Job drawing, mm, ordinate dimensions from the low corner. One solid piece. A direction names the side the tool comes from. Give positions to 0.01 mm unless a question says otherwise; leave off trailing zeros. Write each loop counter-clockwise with the first axis right and the second up, starting at its lowest first coordinate (ties: lowest second). Pieces come first, ordered by that corner, then holes. Notation, with made-up numbers: (76.5, 86.25) - (105.5, 86.25) arc R21 ccw to (105.5, 124.25) - close; hole circle Ø10 at (-31.5, 74). An arc over 180 degrees is marked (long way). Answer as a JSON object with one key per item and string values.
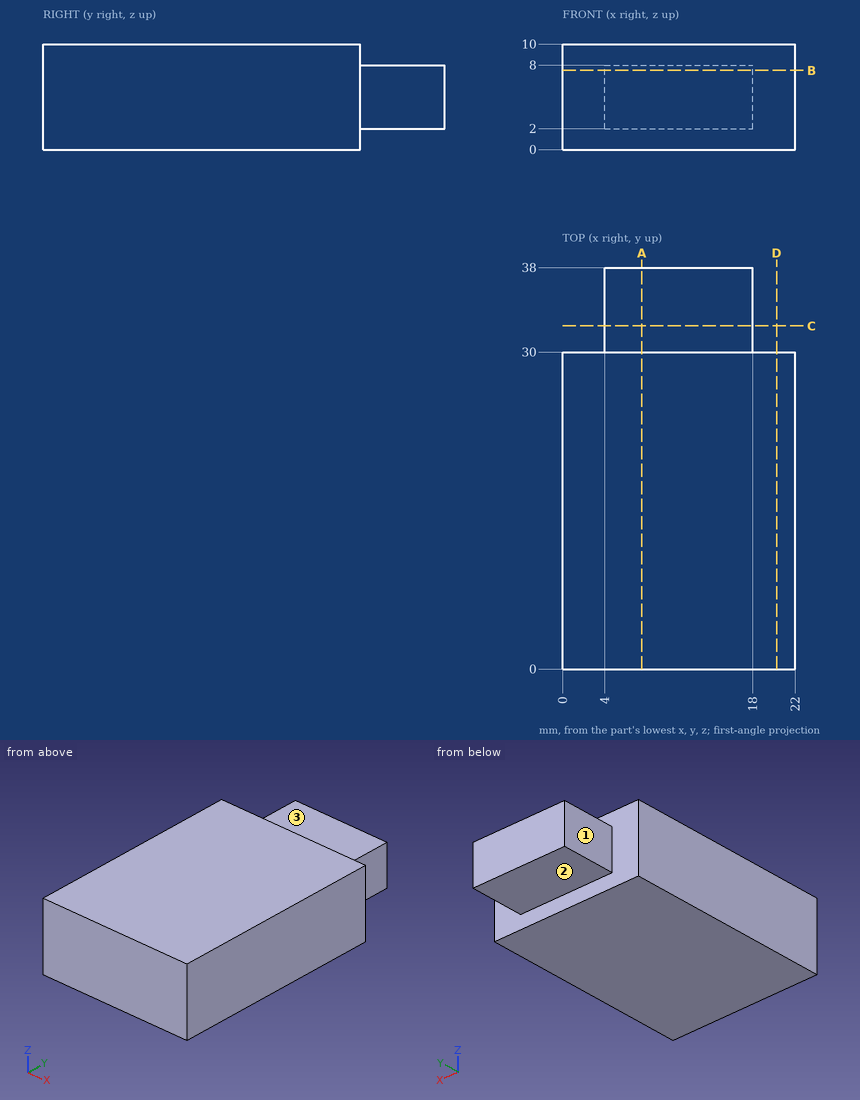
Item 1: Cut at D-D (x = 20.25). Give the cut face in (y, z).
Entries:
{"outline": "(0, 0) - (30, 0) - (30, 10) - (0, 10) - close"}
Item 2: Probe line 1 (Z direction, x = 12, y = 33); line 2 (Y direction, x = 3, z = 3); line 3 (X direction, y = 35, z = 7.75). List the from-to ranges inside material, lowest first. Write a range as from..to.
Entries:
{"line 1": "2..8", "line 2": "0..30", "line 3": "4..18"}
Item 3: Cut at A-A (x = 7.5). Give the cut face in (y, z), and give its area (3 significant figures).
Entries:
{"outline": "(0, 0) - (30, 0) - (30, 2) - (38, 2) - (38, 8) - (30, 8) - (30, 10) - (0, 10) - close", "area": "348 mm2"}
Item 4: Cut at B-B (z = 7.5). Give the cut face in (x, y), and give its area (3 significant figures).
Entries:
{"outline": "(0, 0) - (22, 0) - (22, 30) - (18, 30) - (18, 38) - (4, 38) - (4, 30) - (0, 30) - close", "area": "772 mm2"}
Item 5: Which spindle directions (+Z, -Z, +X, -X, +Y, -Y) get a long thin tool onto all of the face, cutting with end or side? Do the marked faces 1, 2 and 3. Say none if no direction does.
Entries:
{"face 1": "+Z, -Z, -X, +Y", "face 2": "-Z, +X, -X, +Y", "face 3": "+Z, +X, -X, +Y"}
Item 6: Flat gauge pins, fed straight in: P1, Ø3, axis at y = 32.5, z = 3.5, coming from the -X side; P2, Ø2.5, axis at x = 8, y = 35, coming from the +Z side; P3, Ø3, axis at y = 33.5, z = 5.5, coming from the +X side. Where does each tip first touch, or does it go through?
Entries:
{"P1": "x = 4", "P2": "z = 8", "P3": "x = 18"}
Item 7: Cut at C-C (y = 32.5). Give the cut face in (x, z).
Entries:
{"outline": "(4, 2) - (18, 2) - (18, 8) - (4, 8) - close"}
